from build123d import *

# Parameters (mm, degrees)
BOSS_EXTRUDE1_DEPTH = 1.524


with BuildPart() as part:
    # Sketch1 → Boss-Extrude1 (new body)
    with BuildSketch(Plane.XY):
        with BuildLine():
            Line((0.762804565, 0.707113294), (0.762617378, -1.952243646))
            ThreePointArc((0.762617378, -1.952243646), (1.688876918, -2.090003107), (2.330283806, -2.772301873))
            ThreePointArc((2.330283806, -2.772301873), (2.864179893, -5.162377967), (2.419859411, -7.570715168))
            ThreePointArc((2.419859411, -7.570715168), (1.838969345, -9.764772757), (2.419550535, -11.958912099))
            ThreePointArc((2.419550535, -11.958912099), (3.056385936, -10.009011099), (4.324266146, -8.396512102))
            ThreePointArc((4.324266146, -8.396512102), (5.30756259, -5.77657732), (5.883862124, -3.038181986))
            ThreePointArc((5.883862124, -3.038181986), (6.501160971, 0.344941452), (7.217868451, 3.708408777))
            ThreePointArc((7.217868451, 3.708408777), (6.634279276, 2.828156935), (5.838122451, 2.134216059))
            ThreePointArc((5.838122451, 2.134216059), (5.505397312, 3.813158809), (5.018716283, 5.454102548))
            ThreePointArc((5.018716283, 5.454102548), (2.851221099, 9.229151646), (0.000807633, 12.519162913))
            ThreePointArc((0.000807633, 12.519162913), (-2.849605833, 9.229151646), (-5.017101017, 5.454102548))
            ThreePointArc((-5.017101017, 5.454102548), (-5.503782046, 3.813158809), (-5.836507185, 2.134216059))
            ThreePointArc((-5.836507185, 2.134216059), (-6.63266401, 2.828156935), (-7.216253185, 3.708408777))
            ThreePointArc((-7.216253185, 3.708408777), (-6.499545704, 0.344941452), (-5.882246858, -3.038181986))
            ThreePointArc((-5.882246858, -3.038181986), (-5.305947324, -5.77657732), (-4.32265088, -8.396512102))
            ThreePointArc((-4.32265088, -8.396512102), (-3.05477067, -10.009011099), (-2.417935269, -11.958912099))
            ThreePointArc((-2.417935269, -11.958912099), (-1.837354079, -9.764772757), (-2.418244145, -7.570715168))
            ThreePointArc((-2.418244145, -7.570715168), (-2.862564627, -5.162377967), (-2.32866854, -2.772301873))
            ThreePointArc((-2.32866854, -2.772301873), (-1.688352617, -2.090574399), (-0.763422707, -1.951788625))
            Line((-0.763422707, -1.951788625), (-0.761189299, 0.707113294))
            Line((-0.761189299, 0.707113294), (0.762804565, 0.707113294))
        make_face()
    extrude(amount=BOSS_EXTRUDE1_DEPTH)


solid = part.part
Read the model definition and answer for the solid it produces. Units are mm, in the model's axes. A direction names the side the tool comes from. Give positions to 0.01 mm unless a question says otherwise; leave off trailing zeros. Loops run counter-clockwise (first coordinate to the right, second up) from the corner with the lowest first, then second, coordinate; pieces in that order, holes last. Notation, with made-up numbers: (50.5, -16) -> (65.5, -16) arc R33 cw to (65.5, 15) -> close; hole circle Ø1 at (51, 17). An arc over 180 degrees is marked (long way). Use a Markdown table: item, result.
Q1. Section D-D, the plane x = 4.75 is taken. Determine the outline of the cut face in (y, z), then the cut area to 3 significant figures.
Solved:
| item | result |
|---|---|
| outline | (-7.41, 0) -> (6.03, 0) -> (6.03, 1.52) -> (-7.41, 1.52) -> close |
| area | 20.5 mm^2 |
Q2. Determine the mould class of faces 1 (the face through (2.863, -5.128, 0.751)), 2 (the face through (-2.863, -5.197, 0.751)), 3 (the face through (0, 3, 0)), 4 (the face through (6.492, 0.298, 0.751)) for opening direction Y: pulls with the +Y half, pulls with the -Y half, needs draft (parallel to the pull), parting line crosses it, or undercut.
Solved:
| item | result |
|---|---|
| face 1 | undercut |
| face 2 | undercut |
| face 3 | needs draft |
| face 4 | pulls with the -Y half |
Q3. Section B-B, the plane y = -9.5 is taken. Determine the outline of the cut face in (x, z).
Solved:
| item | result |
|---|---|
| outline | (-3.36, 0) -> (-1.85, 0) -> (-1.85, 1.52) -> (-3.36, 1.52) -> close; (1.85, 0) -> (3.36, 0) -> (3.36, 1.52) -> (1.85, 1.52) -> close |
Q4. Section A-A, the plane z = 0.55 is taken. Determine the outline of the cut face in (x, y).
Solved:
| item | result |
|---|---|
| outline | (-7.22, 3.71) arc R116.71 cw to (-5.88, -3.04) arc R18.47 ccw to (-4.32, -8.4) arc R5.88 cw to (-2.42, -11.96) arc R4.44 ccw to (-2.42, -7.57) arc R6.13 cw to (-2.33, -2.77) arc R1.43 cw to (-0.76, -1.95) -> (-0.76, 0.71) -> (0.76, 0.71) -> (0.76, -1.95) arc R1.43 cw to (2.33, -2.77) arc R6.13 cw to (2.42, -7.57) arc R4.44 ccw to (2.42, -11.96) arc R5.88 cw to (4.32, -8.4) arc R18.47 ccw to (5.88, -3.04) arc R116.71 cw to (7.22, 3.71) arc R3.95 cw to (5.84, 2.13) arc R18.47 ccw to (5.02, 5.45) arc R22.62 ccw to (0, 12.52) arc R22.62 ccw to (-5.02, 5.45) arc R18.47 ccw to (-5.84, 2.13) arc R3.95 cw to start |
Q5. Section C-C, the plane y = -4.5 is taken. Determine the outline of the cut face in (x, z).
Solved:
| item | result |
|---|---|
| outline | (-5.63, 0) -> (-2.81, 0) -> (-2.81, 1.52) -> (-5.63, 1.52) -> close; (2.82, 0) -> (5.63, 0) -> (5.63, 1.52) -> (2.82, 1.52) -> close |
Q6. Find the intervals of material crossed by line 1 along X through (y, z) = (-0.5, 1.2); line 2 along X through (y, z) = (-9.5, 0.2); line 3 along Y through (x, z) = (2.25, 1), in increasing order.
Solved:
| item | result |
|---|---|
| line 1 | x = -6.34 to -0.76, 0.76 to 6.34 |
| line 2 | x = -3.36 to -1.85, 1.85 to 3.36 |
| line 3 | y = -11.63 to -7.9, -2.62 to 10.04 |
Q7. A tool of negligible diameter and unlimited length cuts with its end or side. For faces 5 (the face through (0, 0.707, 1)), 6 (the face through (-5.317, -5.739, 0.751)), 7 (the face through (-1.837, -9.797, 0.751)), from which of +Z, -Z, +X, -X, +Y, -Y can it reach the whole face along a straight path? Write none if from no direction.
Solved:
| item | result |
|---|---|
| face 5 | +Z, -Z, -Y |
| face 6 | +Z, -Z, -X, -Y |
| face 7 | +Z, -Z |
